```python
from build123d import *

# Parameters (mm, degrees)
BOSS_EXTRUDE1_DEPTH = 38.1
SKETCH2_R           = 3.175
BOSS_EXTRUDE2_DEPTH = 48.26
FILLET1_R           = 19.05


with BuildPart() as part:
    # Sketch1 → Boss-Extrude1 (new body)
    with BuildSketch(Plane(origin=(0, 0, 0), x_dir=(1, 0, 0), z_dir=(0, 1, 0))):
        with BuildLine():
            Line((-3.175, 0), (-3.175, 114.3))
            ThreePointArc((-3.175, 114.3), (0, 117.475), (3.175, 114.3))
            Line((3.175, 114.3), (3.175, 1.884785088))
            Line((3.175, 1.884785088), (71.370355515, -35.312681556))
            ThreePointArc((71.370355515, -35.312681556), (72.637318444, -39.620355515), (68.329644485, -40.887318444))
            Line((68.329644485, -40.887318444), (-1.520355515, -2.787318444))
            ThreePointArc((-1.520355515, -2.787318444), (-2.73017891, -1.620724566), (-3.175, 0))
        make_face()
    extrude(amount=BOSS_EXTRUDE1_DEPTH)

    # Sketch2 → Boss-Extrude2 (add)
    with BuildSketch(Plane(origin=(0, 0, 0), x_dir=(-1, 0, 0), z_dir=(0, -1, 0))):
        with Locations(Location((0, 114.3, 0), (0, 0, 90))):
            Circle(SKETCH2_R)
        with Locations(Location((0, 0, 0), (0, 0, 90))):
            Circle(SKETCH2_R)
        with Locations(Location((-69.85, -38.1, 0), (0, 0, 90))):
            Circle(SKETCH2_R)
    extrude(amount=-BOSS_EXTRUDE2_DEPTH)

    # Fillet1
    fillet1_edges = [part.edges().sort_by_distance(p)[0] for p in [
        (3.175, 19.05, -1.884785088),
    ]]
    fillet(fillet1_edges, radius=FILLET1_R)


solid = part.part
```
Check sheet for the modelled part. Datum: model origin and axes. Units: mm. A direction names the side the tool comes from. Give positions to 0.01 mm unless a question says otherwise; leave off trailing zeros. Order: outer loops, then holes, each group sorted by start corner. A loop starts at its lowest first (then second) coordinate and runs counter-clockwise, first axis right, second up. Notation, with made-up numbers: M -25.5,57.25 L 31.5,57.25 A21 ccw 31.5,68.25 Z; hole C 42,-22.5 d8. An arc over 180 degrees is marked long. Answer in a Markdown table with one row per item.
1) Cross-section at C-C, the plane x = 69.85. Enter the section's corners in (y, z) (3 decimals).
Filled sheet:
| item | result |
|---|---|
| outline | M 0,34.483 L 38.1,34.483 L 38.1,34.925 L 48.26,34.925 L 48.26,41.275 L 0,41.275 Z |
2) Cross-section at D-D, the plane z = -98. Enter the section's corners in (x, y) (3 decimals).
Filled sheet:
| item | result |
|---|---|
| outline | M -3.175,0 L 3.175,0 L 3.175,38.1 L -3.175,38.1 Z |
3) Access from +Z, -Z, +X, -X, +Y, -Y to the whole of each face (thin tool, end or side, straight path). Record for faces 1 (the flat face through (0, 48.26, 0)), 2 (the cylindrical face through (71.996, 29.154, 40.44)), 3 (the flat face through (3.175, 19, -64)).
Filled sheet:
| item | result |
|---|---|
| face 1 | +Z, -Z, +X, -X, +Y |
| face 2 | +Y |
| face 3 | -Z, +X, +Y, -Y |
4) Gauge pin test, flat ends, axial feed: P1, Ø3, axis at y = 19, z = -100.5, coming from the +X side (3 decimals); P2, Ø10, axis at x = 65, z = 25, coming from the +Y side (3 decimals); P3, Ø1.5, axis at x = 57.5, y = 32.5, coming from the -Z side; P4, Ø5, axis at x = 10, y = 18.5, coming from the +Z side. Record the tip position at first contact, or that the pin passes through.
Filled sheet:
| item | result |
|---|---|
| P1 | stops at x = 3.175 |
| P2 | passes through |
| P3 | stops at z = 27.34 |
| P4 | stops at z = 10.43 |
5) Cross-section at B-B, the plane y = 41. Enter the section's corners in (x, z) (3 decimals).
Filled sheet:
| item | result |
|---|---|
| outline | C 0,-114.3 d6.35; C 0,0 d6.35; C 69.85,38.1 d6.35 |
6) Thickness scan on L1, parallel to X at y = 31.5, z = -95.5 (3 decimals); L2, parallel to Y at x = 7, z = -1; L3, parallel to Z at x = 9, y = 18. Record the ranges inside material, lowest first. Write a range as [from, to].
Filled sheet:
| item | result |
|---|---|
| L1 | x = [-3.175, 3.175] |
| L2 | y = [0, 38.1] |
| L3 | z = [0.52, 8.53] |
7) Release check for a two-part mould opening along Z. For faces 4 (the flat face through (33.89, 18.78, 22.1)), 5 (the flat face through (1, 0, -27)), 6 (the flat face through (1, 38.1, -20)) record: +Z half, -Z half, draft (parallel to the pull), parting line (faces both ways), or undercut.
Filled sheet:
| item | result |
|---|---|
| face 4 | +Z half |
| face 5 | draft |
| face 6 | undercut |
